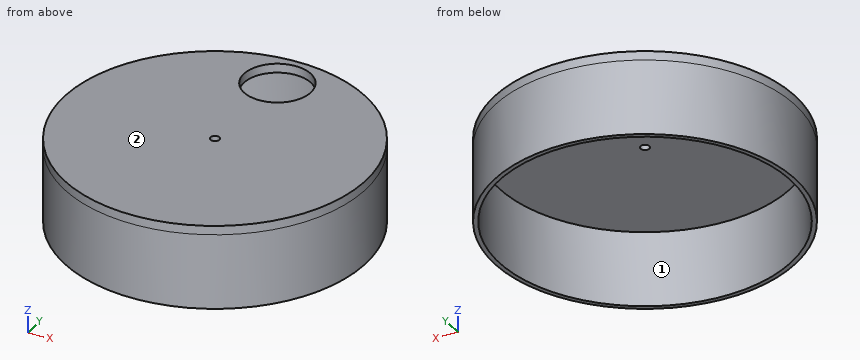
from build123d import *

# Parameters (mm, degrees)
SKETCH1_R           = 100
BOSS_EXTRUDE1_DEPTH = 6
BOSS_EXTRUDE2_START = 50
SKETCH2_R           = 100
SKETCH2_R_2         = 97
BOSS_EXTRUDE2_DEPTH = 50
SKETCH4_R           = 22.225
CUT_EXTRUDE2_DEPTH  = 50
SKETCH5_R           = 3
CUT_EXTRUDE3_DEPTH  = 50


with BuildPart() as part:
    # Sketch1 → Boss-Extrude1 (new body)
    with BuildSketch(Plane.XY):
        Circle(SKETCH1_R)
    extrude(amount=BOSS_EXTRUDE1_DEPTH)

    # Sketch2 → Boss-Extrude2 (add)
    with BuildSketch(Plane(origin=(0, 0, 0), x_dir=(-1, 0, 0), z_dir=(0, 0, -1)).offset(BOSS_EXTRUDE2_START)):
        Circle(SKETCH2_R)
        Circle(SKETCH2_R_2, mode=Mode.SUBTRACT)
    extrude(amount=-BOSS_EXTRUDE2_DEPTH)

    # Sketch4 → Cut-Extrude2 (cut)
    with BuildSketch(Plane(origin=(0, 0, 0), x_dir=(-1, 0, 0), z_dir=(0, 0, -1))):
        with Locations((0, 73)):
            Circle(SKETCH4_R)
    extrude(amount=-CUT_EXTRUDE2_DEPTH, mode=Mode.SUBTRACT)

    # Sketch5 → Cut-Extrude3 (cut)
    with BuildSketch(Plane(origin=(0, 0, 0), x_dir=(-1, 0, 0), z_dir=(0, 0, -1))):
        Circle(SKETCH5_R)
    extrude(amount=-CUT_EXTRUDE3_DEPTH, mode=Mode.SUBTRACT)


solid = part.part
Input: part model. Units: mm. Frame: model coordinates. Face numbers are marked on the shaded views. Coordinates: 2 decimals unless noted, no trailing zeros. Loops run counter-clockwise (first coordinate to the right, second up) from the corner with the lowest first, then second, coordinate; pieces in that order, holes last. Notation, with made-up numbers: (-19, -5.75) -> (32, -5.75) arc R13 ccw to (32, 12.25) -> close; hole circle Ø11 at (-39.5, 35). An arc over 180 degrees is marked (long way). One line per item, written item: value.
(1) Pin query (flat end, axial travel): pin 1 Ø10 at (y, z) = (43, -33.5) entering from -X; pin 2 Ø6 at (y, z) = (64.5, -35) entering from -X; pin 3 Ø3 at (y, z) = (7, -26) entering from -X; pin 4 Ø3.5 at (x, y) = (0, 0) entering from +Z. Return the tip coordinate at first contact, or that it passes through.
Answer below:
pin 1: stops at x = -92.5
pin 2: stops at x = -78.85
pin 3: stops at x = -99.85
pin 4: passes through
(2) Draft query along Y for the marked faces 1 and 2. Return one class per face: pulls with the +Y half, pulls with the -Y half, needs draft (parallel to the pull), parting line crosses it, or undercut.
Answer below:
face 1: undercut
face 2: needs draft
(3) Cut plane C-C (y = -65). Output: boundary loops of the cut face in (x, z), then the cut area to 3 significant figures.
Answer below:
outline: (-75.99, -50) -> (-72, -50) -> (-72, 0) -> (72, 0) -> (72, -50) -> (75.99, -50) -> (75.99, 6) -> (-75.99, 6) -> close
area: 1,310 mm2
(4) Cut plane A-A (y = 0). Output: boundary loops of the cut face in (x, z), then the cut area to 3 significant figures.
Answer below:
outline: (-100, -50) -> (-97, -50) -> (-97, 0) -> (-3, 0) -> (-3, 6) -> (-100, 6) -> close; (3, 0) -> (97, 0) -> (97, -50) -> (100, -50) -> (100, 6) -> (3, 6) -> close
area: 1,460 mm2
(5) Cut plane B-B (x = 0). Output: boundary loops of the cut face in (y, z) (3 decimals).
Answer below:
outline: (-100, -50) -> (-97, -50) -> (-97, 0) -> (-3, 0) -> (-3, 6) -> (-100, 6) -> close; (3, 0) -> (50.775, 0) -> (50.775, 6) -> (3, 6) -> close; (95.225, 0) -> (97, 0) -> (97, -50) -> (100, -50) -> (100, 6) -> (95.225, 6) -> close
(6) Cut plane D-D (z = -41). Output: boundary loops of the cut face in (x, y).
Answer below:
outline: circle Ø200 at (0, 0); hole circle Ø194 at (0, 0)
(7) Ray query, line 1 along Y through (x, z) = (0, 2) (3 decimals); line 2 along Z through (x, y) = (11, -10); line 3 along X through (y, z) = (33.5, -12). Return the intervals inside material, ascending.
Answer below:
line 1: y = -100 to -3, 3 to 50.775, 95.225 to 100
line 2: z = 0 to 6
line 3: x = -94.22 to -91.03, 91.03 to 94.22
